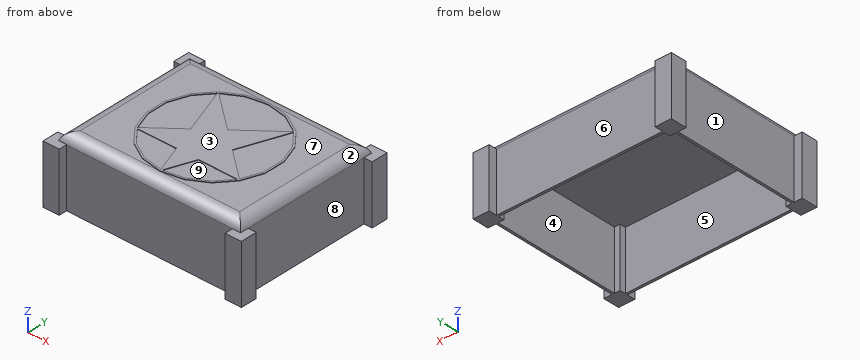
```python
from build123d import *

# Parameters (mm, degrees)
F0_W        = 77.5
F0_H        = 61
F1_DEPTH    = 3.5
F2_T1_DEPTH = 84.8484800354
F2_T3_DEPTH = 101.3484800354
F5_DEPTH    = 25
F6_DEPTH    = 0.2


# Not quite as in the source:
# - a fillet or chamfer that OpenCascade refuses, or shapes differently, is made with other operations: its cross-section is extruded or revolved along the edge and cut away or added


with BuildPart() as f1:
    # F0 (on Top) → F1 (new body)
    with BuildSketch(Plane.XY):
        Rectangle(F0_W, F0_H)
    extrude(amount=F1_DEPTH)

    # F2: fillet of radius 5 on 4 edges, made by hand

    # F2_s2 → F2_t1 (cut)
    with BuildSketch(Plane.XZ.offset(-42.4242400177)):
        with BuildLine():
            ThreePointArc((38.75, 0), (36.9383438845, 2.5311288741), (33.9803039929, 3.5))
            Line((33.9803039929, 3.5), (38.75, 3.5))
            Line((38.75, 3.5), (38.75, 0))
        make_face()
        with BuildLine():
            ThreePointArc((-38.75, 0), (-36.9383438845, 2.5311288741), (-33.9803039929, 3.5))
            Line((-33.9803039929, 3.5), (-38.75, 3.5))
            Line((-38.75, 3.5), (-38.75, 0))
        make_face()
    extrude(amount=F2_T1_DEPTH, mode=Mode.SUBTRACT)

    # F2_s4 → F2_t3 (cut)
    with BuildSketch(Plane.YZ.offset(-50.6742400177)):
        with BuildLine():
            ThreePointArc((30.5, 0), (28.6883438845, 2.5311288741), (25.7303039929, 3.5))
            Line((25.7303039929, 3.5), (30.5, 3.5))
            Line((30.5, 3.5), (30.5, 0))
        make_face()
        with BuildLine():
            ThreePointArc((-30.5, 0), (-28.6883438845, 2.5311288741), (-25.7303039929, 3.5))
            Line((-25.7303039929, 3.5), (-30.5, 3.5))
            Line((-30.5, 3.5), (-30.5, 0))
        make_face()
    extrude(amount=F2_T3_DEPTH, mode=Mode.SUBTRACT)

    # F4 (on face) → F5 (join)
    with BuildSketch(Plane(origin=(0, 0, 0), x_dir=(1, 0, 0), z_dir=(0, 0, -1))):
        Polygon((-38.75, 29.5), (-38.75, 30.5), (-37.75, 30.5), (-35.3, 30.5), (-35.3, 33.95), (-42.2, 33.95), (-42.2, 27.05), (-38.75, 27.05), align=None)
        Polygon((-37.75, 30.5), (-38.75, 30.5), (-38.75, 29.5), (-38.75, 27.05), (-38.75, -27.05), (-38.75, -29.5), (-38.75, -30.5), (-37.75, -30.5), (-35.3, -30.5), (35.3, -30.5), (37.75, -30.5), (38.75, -30.5), (38.75, -29.5), (38.75, -27.05), (38.75, 27.05), (38.75, 29.5), (38.75, 30.5), (37.75, 30.5), (35.3, 30.5), (-35.3, 30.5), align=None)
        Polygon((-35.3, 27.05), (-35.3, 29.5), (35.3, 29.5), (35.3, 27.05), (37.75, 27.05), (37.75, -27.05), (35.3, -27.05), (35.3, -29.5), (-35.3, -29.5), (-35.3, -27.05), (-37.75, -27.05), (-37.75, 27.05), align=None, mode=Mode.SUBTRACT)
        Polygon((35.3, 33.95), (35.3, 30.5), (37.75, 30.5), (38.75, 30.5), (38.75, 29.5), (38.75, 27.05), (42.2, 27.05), (42.2, 33.95), align=None)
        Polygon((-38.75, -29.5), (-38.75, -27.05), (-42.2, -27.05), (-42.2, -33.95), (-35.3, -33.95), (-35.3, -30.5), (-37.75, -30.5), (-38.75, -30.5), align=None)
        Polygon((42.2, -27.05), (38.75, -27.05), (38.75, -29.5), (38.75, -30.5), (37.75, -30.5), (35.3, -30.5), (35.3, -33.95), (42.2, -33.95), align=None)
    extrude(amount=F5_DEPTH)

    # F3 (on face) → F6 (join)
    with BuildSketch(Plane.XY.offset(3.5)):
        Polygon((-16.2400073105, 18.8887493843), (-8.7504151188, -1.6887360431), (0.1768791019, 5.6841672089), (-15.9216975961, 19.1924769786), (-16.0447749761, 19.1214182202), align=None)
        Polygon((-21.294405657, -12.8651519965), (-4.682532386, -12.8651519965), (-8.7504151188, -1.6887360431), (-21.6633903185, -12.3533466729), (-21.6170668475, -12.4806193635), align=None)
        Polygon((-4.682532386, -12.8651519965), (-0.2991132897, -24.9084969837), (0, -24.961238727), (0.3027663667, -24.9078528477), (4.7360081498, -12.8651519965), align=None)
        Polygon((8.8770657691, -1.6161562148), (4.7360081498, -12.8651519965), (21.294405657, -12.8651519965), (21.6170668475, -12.4806193635), (21.665673901, -12.3470725815), align=None)
        Polygon((0.1768791019, 5.6841672089), (8.8770657691, -1.6161562148), (16.3689174848, 18.7351202209), (16.20943331, 18.9251860592), align=None)
        Polygon((-25.3394028596, -4.4680203992), (-22.283096905, -12.8651519965), (-21.6633903185, -12.3533466729), (-24.5820214231, -4.3344736172), (-24.5820214231, 4.3344736172), (-21.6170668475, 12.4806193635), (-16.2400073105, 18.8887493843), (-16.5391206001, 19.7105563935), (-22.283096905, 12.8651519965), (-25.3394028596, 4.4680203992), align=None)
        Polygon((0.3027663667, -24.9078528477), (0, -25.7303039929), (8.8002822595, -24.1785767927), (16.5391206001, -19.7105563935), (22.283096905, -12.8651519965), (21.294405657, -12.8651519965), (16.0447749761, -19.1214182202), (8.537246447, -23.4558918374), align=None)
        Polygon((-8.8002822595, -24.1785767927), (0, -25.7303039929), (-0.2991132897, -24.9084969837), (-8.537246447, -23.4558918374), (-16.0447749761, -19.1214182202), (-21.294405657, -12.8651519965), (-22.283096905, -12.8651519965), (-16.5391206001, -19.7105563935), align=None)
        Polygon((-22.283096905, -12.8651519965), (-21.294405657, -12.8651519965), (-21.6170668475, -12.4806193635), (-21.6633903185, -12.3533466729), align=None)
        Polygon((-16.5391206001, 19.7105563935), (-16.2400073105, 18.8887493843), (-16.0447749761, 19.1214182202), (-15.9216975961, 19.1924769786), align=None)
        Polygon((21.665673901, -12.3470725815), (22.283096905, -12.8651519965), (25.3394028596, -4.4680203992), (25.3394028596, 4.4680203992), (22.283096905, 12.8651519965), (16.5391206001, 19.7105563935), (8.8002822595, 24.1785767927), (0, 25.7303039929), (-8.8002822595, 24.1785767927), (-16.5391206001, 19.7105563935), (-15.9216975961, 19.1924769786), (-8.537246447, 23.4558918374), (0, 24.961238727), (8.537246447, 23.4558918374), (16.0447749761, 19.1214182202), (16.20943331, 18.9251860592), (16.5391206001, 19.1974692878), (16.3689174848, 18.7351202209), (21.6170668475, 12.4806193635), (24.5820214231, 4.3344736172), (24.5820214231, -4.3344736172), align=None)
        Polygon((16.20943331, 18.9251860592), (16.3689174848, 18.7351202209), (16.5391206001, 19.1974692878), align=None)
        Polygon((21.6170668475, -12.4806193635), (21.294405657, -12.8651519965), (22.283096905, -12.8651519965), (21.665673901, -12.3470725815), align=None)
        Polygon((-0.2991132897, -24.9084969837), (0, -25.7303039929), (0.3027663667, -24.9078528477), (0, -24.961238727), align=None)
        Polygon((-8.7504151188, -1.6887360431), (-4.682532386, -12.8651519965), (4.7360081498, -12.8651519965), (8.8770657691, -1.6161562148), (0.1768791019, 5.6841672089), align=None)
    extrude(amount=F6_DEPTH)


solid = f1.part
```
Geometry check sheet. Reference: the model listing, model coordinates, mm. Face numbers are marked on the shaded views. A direction names the side the tool comes from. Round coordinates to 2 decimals unless told otherwise and drop trailing zeros. Loops run counter-clockwise (first coordinate to the right, second up) from the corner with the lowest first, then second, coordinate; pieces in that order, holes last. Notation, with made-up numbers: (59.5, 58.5) - (78.5, 58.5) arc R7 cw to (78.5, 64.5) - close; hole circle Ø11 at (38.5, 28.25). An arc over 180 degrees is marked (long way). Write item = value, one per line. Start each with the question number.
1. Section check B-B on x = -32.5. Enter the section's corners in (y, z).
2. Section check D-D on y = -22.5. Enter the section's corners in (x, z).
3. Depth check by flat-ended pin: pin 1 (12.5 mm diameter, centred on y = -7, z = -13, fed in from +X); pin 2 (7.5 mm diameter, centred on x = -13, z = -10.5, fed in from -Y); pin 3 (7.5 mm diameter, centred on x = -11, z = -7, fed in from +Y). Enter the tip coordinate at first touch or a pass-through.
4. Section check C-C on y = -14.5. Enter the section's corners in (x, z), then the cut area to 3 significant figures.
5. Thickness scan on line 1 (Y direction, x = -13.5, z = -6); line 2 (X direction, y = 4, z = -14.5); line 3 (Z direction, x = -23, y = -26). Record the ranges inside material, lowest first.
6. Mould release check, pull along X, two halves, no side actions. Record for the marked faces 1, 2, 3 and 4: released by +X, released by -X, zero draft, split by the parting line, or undercut.
7. Set-up check for the marked faces 5, 6, 7, 8 and 9: record each of +Z, -Z, +X, -X, +Y, -Y from which the full face is reachable in a straight line by a thin tool's end or side.
Working result:
q1.outline = (-30.5, -25) - (-29.5, -25) - (-29.5, 0) - (29.5, 0) - (29.5, -25) - (30.5, -25) - (30.5, 0) arc R5 ccw to (25.73, 3.5) - (-25.73, 3.5) arc R5 ccw to (-30.5, 0) - close
q2.outline = (-38.75, -25) - (-37.75, -25) - (-37.75, 0) - (37.75, 0) - (37.75, -25) - (38.75, -25) - (38.75, 0) arc R5 ccw to (33.98, 3.5) - (11.71, 3.5) - (11.71, 3.7) - (10.19, 3.7) - (10.19, 3.5) - (1.19, 3.5) - (1.19, 3.7) - (-1.18, 3.7) - (-1.18, 3.5) - (-10.19, 3.5) - (-10.19, 3.7) - (-11.71, 3.7) - (-11.71, 3.5) - (-33.98, 3.5) arc R5 ccw to (-38.75, 0) - close
q3.pin_1 = 38.75
q3.pin_2 = -30.5
q3.pin_3 = 30.5
q4.outline = (-38.75, -25) - (-37.75, -25) - (-37.75, 0) - (37.75, 0) - (37.75, -25) - (38.75, -25) - (38.75, 0) arc R5 ccw to (33.98, 3.5) - (20.91, 3.5) - (20.91, 3.7) - (19.92, 3.7) - (19.92, 3.5) - (4.13, 3.5) - (4.13, 3.7) - (-4.09, 3.7) - (-4.09, 3.5) - (-19.92, 3.5) - (-19.92, 3.7) - (-20.91, 3.7) - (-20.91, 3.5) - (-33.98, 3.5) arc R5 ccw to (-38.75, 0) - close
q4.area = 314 mm^2
q5.line_1 = -30.5 to -29.5, 29.5 to 30.5
q5.line_2 = -38.75 to -37.75, 37.75 to 38.75
q5.line_3 = 0 to 3.49
q6.face_1 = released by -X
q6.face_2 = released by +X
q6.face_3 = zero draft
q6.face_4 = undercut
q7.face_5 = -Z
q7.face_6 = +Z, -Z, +Y
q7.face_7 = +Z, +X
q7.face_8 = +Z, -Z, +X
q7.face_9 = +Z
